Verification items for the finished model (mm, model axes). A direction names the side the tool comes from. Give positions to 0.01 mm unless a question says otherwise; leave off trailing zeros. Order: outer loops, then holes, each group sorted by start corner. A loop starts at its lowest first (then second) coordinate and runs counter-clockwise, first axis right, second up. Notation, with made-up numbers: (43, -14.75) -> (85, -14.75) arc R24 ccw to (85, 23.25) -> close; hole circle Ø8 at (35, -16). An arc over 180 degrees is marked (long way). One line per question, with ' | ' between items. Start each with the question number.
Q1. Material ranges on probe 1 along Y at (x, z) = (2, 14.5); probe 2 along Y at (x, z) = (-16.5, 16); probe 3 along X at (y, z) = (-9, -34), recorded low to high. Write a range as [from, to].
Q2. Mould release check, pull along Y, two halves, no side actions. Record for faces 3 (the conical face through (-4.245, 19.117, -7.048)), 4 (the flat face through (8.5, -5, 2)), 5 (the flat face through (-0.3, 0.3, 20)): released by +Y, released by -Y, zero draft, split by the parting line, or undercut.
Q3. Section check A-A on z = 8.5. Record the cut outline in (x, y), plus the area to 3 significant figures.
Q4. Go/stop test with flat-tipped pins: pin 1 (1.5 mm diameter, centred on y = -3, z = -29, fed in from -X); pin 2 (3 mm diameter, centred on x = -13, y = 1.5, fed in from -Z); pin 3 (8 mm diameter, centred on x = 2, z = -8, fed in from +Y). Record where each tip stops, or that it passes through.
Q5. Access from +Z, -Z, +X, -X, +Y, -Y to the whole of each face (thin tool, end or side, straight path). Record for faces 1 (the flat face through (0, -14.864, 5)), 2 (the flat face through (0, -2, -10)).
Q6. Section check B-B on z = -11. Record the cut outline in (x, y), plus the area to 3 significant figures.
from build123d import *

# Parameters (mm, degrees)
SKETCH_4_W          = 17
SKETCH_4_H          = 15
CUT_EXTRUDE_1_DEPTH = 30
SKETCH_5_W          = 17
SKETCH_5_H          = 12
CUT_EXTRUDE_2_DEPTH = 25


with BuildPart() as part:
    # Sketch 1 → Revolve 1 (revolve)
    with BuildSketch(Plane(origin=(0, 0, 0), x_dir=(1, 0, 0), z_dir=(0, 1, 0)), mode=Mode.PRIVATE) as revolve_1_sk:
        with BuildLine():
            Line((-21, -20), (0, -20))
            Line((0, -20), (0, 76.509456591))
            add(Edge.make_bspline(
                [(-21, 23.303526799), (-20.950151988, 23.55619715), (-20.588242456, 25.356689417), (-19.861805291, 28.542980585), (-18.781007648, 32.618309393), (-17.683803917, 36.387694686), (-16.794111183, 39.324775715), (-16.139995318, 41.546015667), (-15.635538449, 43.197589032), (-15.024163935, 45.012380328), (-13.937228163, 47.886209516), (-11.955046686, 52.531179902), (-8.996626021, 58.945239937), (-6.340494309, 64.415530495), (-4.283171781, 68.509695264), (-2.81904039, 71.351111958), (-1.479938004, 73.873249362), (-0.567336195, 75.524317414), (-0.112134261, 76.316693352), (0, 76.509456591)],
                knots=[0.246223276, 0.246223276, 0.246223276, 0.246223276, 0.255865129, 0.31540599, 0.374946852, 0.434487714, 0.494028576, 0.523799007, 0.553569438, 0.583339868, 0.613110299, 0.672651161, 0.732192023, 0.791732885, 0.821503316, 0.851273747, 0.881044177, 0.910814608, 0.921120543, 0.921120543, 0.921120543, 0.921120543], degree=3))
            Line((-21, 23.303526799), (-21, -20))
        make_face()
    revolve(revolve_1_sk.sketch.rotate(Axis((0, 0, -76.509456591), (0, 0, 1)), 180), axis=Axis((0, 0, -76.509456591), (0, 0, 1)))

    # Sketch 2 → Cut-Revolve 1 (revolve, cut)
    with BuildSketch(Plane(origin=(0, 0, 0), x_dir=(1, 0, 0), z_dir=(0, 1, 0))):
        Polygon((21, -20), (21, 66.971973821), (16.441991992, 66.971973821), align=None)
    revolve(axis=Axis((0, 0, 20), (0, 0, -1)), mode=Mode.SUBTRACT)

    # Sketch 3 → Cut-Revolve 2 (revolve, cut)
    with BuildSketch(Plane(origin=(0, 0, 0), x_dir=(1, 0, 0), z_dir=(0, 1, 0))):
        with BuildLine():
            Line((1e-08, 76.509474859), (1e-08, 74.388246536))
            ThreePointArc((1e-08, 74.388246536), (1.026734817, 74.10458439), (1.762223825, 73.334062167))
            Line((1.762223825, 73.334062167), (4.025925166, 73.334062167))
            Line((4.025925166, 73.334062167), (4.025925166, 76.509474859))
            Line((4.025925166, 76.509474859), (1e-08, 76.509474859))
        make_face()
    revolve(axis=Axis((1e-08, 0, -76.509474859), (0, 0, 1)), mode=Mode.SUBTRACT)

    # Sketch 4 → Cut-Extrude 1 (cut)
    with BuildSketch(Plane.XY.offset(20)):
        with Locations((0, -7.363542794)):
            Rectangle(SKETCH_4_W, SKETCH_4_H)
    extrude(amount=-CUT_EXTRUDE_1_DEPTH, mode=Mode.SUBTRACT)

    # Sketch 5 → Cut-Extrude 2 (cut)
    with BuildSketch(Plane(origin=(0, -14.863542794, 0), x_dir=(1, 0, 0), z_dir=(0, 1, 0))):
        with Locations((0, 4)):
            Rectangle(SKETCH_5_W, SKETCH_5_H)
    extrude(amount=CUT_EXTRUDE_2_DEPTH, mode=Mode.SUBTRACT)


solid = part.part
Filled in:
1) probe 1: [-20.61, -14.86], [0.14, 20.61] | probe 2: [-12.65, 12.65] | probe 3: [-15.78, 15.78]
2) face 3: split by the parting line | face 4: undercut | face 5: zero draft
3) outline: circle Ø40.79 at (0, 0); hole (-8.5, -14.86) -> (8.5, -14.86) -> (8.5, 0.14) -> (-8.5, 0.14) -> close | area: 1,050 mm²
4) pin 1: x = -18.3 | pin 2: z = -53.28 | pin 3: y = 19.72
5) face 1: +Z | face 2: none
6) outline: circle Ø38.75 at (0, 0) | area: 1,180 mm²
